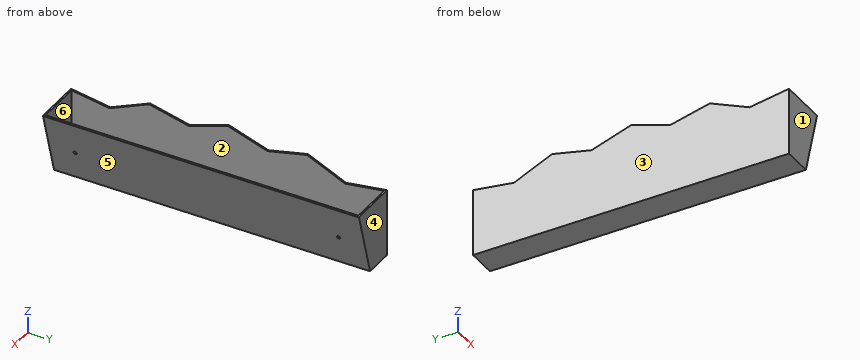
from build123d import *

# Parameters (mm, degrees)
F1_DEPTH  = 304.8
F4_DEPTH  = 1.5875
F6_DEPTH  = 1.5875
F8_DEPTH  = 25.4
F9_DEPTH  = 25.4
F10_DEPTH = 1.5875


with BuildPart() as f1:
    # F0 (on Front) → F1 (new body)
    with BuildSketch(Plane.XZ):
        Polygon((0, 0), (0, 63.5), (-1.5875, 63.5), (-1.5875, -1.5875), (26.5975192948, -1.5875), (45.0656705162, 63.0639608604), (43.5392282085, 63.5), (25.4, 0), align=None)
    extrude(amount=F1_DEPTH)

    # F3 (on face) → F4 (join)
    with BuildSketch(Plane.XZ.offset(304.8)):
        Polygon((43.5392282085, 63.5), (0, 63.5), (0, 0), (25.4, 0), align=None)
    extrude(amount=-F4_DEPTH)

    # F5 (on face) → F6 (join)
    with BuildSketch(Plane(origin=(0, 0, 0), x_dir=(-1, 0, 0), z_dir=(0, 1, 0))):
        Polygon((0, 63.5), (-43.5392282085, 63.5), (-25.4, 0), (0, 0), align=None)
    extrude(amount=-F6_DEPTH)

    # F7 (on face) → F8 (cut)
    with BuildSketch(Plane(origin=(25.0101701183, 0, -7.1443335954), x_dir=(0, 1, 0), z_dir=(0.9615384615, 0, -0.2746703242))):
        with BuildLine():
            ThreePointArc((-279.4, 35.9416069393), (-278.2774679849, 36.4065749241), (-277.8125, 37.5291069393))
            ThreePointArc((-277.8125, 37.5291069393), (-279.4, 39.1166069393), (-280.9875, 37.5291069393))
            ThreePointArc((-280.9875, 37.5291069393), (-280.5225320151, 36.4065749241), (-279.4, 35.9416069393))
        make_face()
        with BuildLine():
            ThreePointArc((-23.8125, 37.5291069393), (-26.5225320151, 38.6516389544), (-25.4, 35.9416069393))
            ThreePointArc((-25.4, 35.9416069393), (-24.2774679849, 36.4065749241), (-23.8125, 37.5291069393))
        make_face()
    extrude(amount=-F8_DEPTH, mode=Mode.SUBTRACT)

    # F2 (on face) → F9 (cut)
    with BuildSketch(Plane.YZ):
        Polygon((-52.2120932715, 63.5), (-39.4870413326, 57.779973409), (-0.1351656424, 63.5), align=None)
        Polygon((-304.8, 63.5), (-266.746729324, 57.5579500411), (-253.1458196474, 63.5), align=None)
    extrude(amount=-F9_DEPTH, mode=Mode.SUBTRACT)

    # F2 (on face) → F10 (join)
    with BuildSketch(Plane.YZ):
        Polygon((-0.1351656424, 63.5), (-39.4870413326, 57.779973409), (0, 63.5), align=None)
        with BuildLine():
            Line((-76.2, 50.6074602206), (0, 50.6074602206))
            ThreePointArc((0, 50.6074602206), (-19.6950538014, 54.4605428278), (-39.4870413326, 57.779973409))
            ThreePointArc((-39.4870413326, 57.779973409), (-57.8141368142, 60.3662538666), (-76.2, 62.4949413282))
            Line((-76.2, 62.4949413282), (-76.2, 50.6074602206))
        make_face()
        with BuildLine():
            Line((-152.4, 50.6074602206), (-76.2, 50.6074602206))
            Line((-76.2, 50.6074602206), (-76.2, 62.4949413282))
            ThreePointArc((-76.2, 62.4949413282), (-81.4321305003, 63.0160017697), (-86.6678194969, 63.5))
            Line((-86.6678194969, 63.5), (-152.4, 63.5))
            Line((-152.4, 63.5), (-152.4, 50.6074602206))
        make_face()
        with BuildLine():
            ThreePointArc((-76.2, 62.4949413282), (-57.8141368142, 60.3662538666), (-39.4870413326, 57.779973409))
            Line((-39.4870413326, 57.779973409), (-52.2120932715, 63.5))
            Line((-52.2120932715, 63.5), (-76.2, 74.2827822634))
            Line((-76.2, 74.2827822634), (-114.3780665248, 65.4410439145))
            ThreePointArc((-114.3780665248, 65.4410439145), (-100.5138654868, 64.6001122426), (-86.6678194969, 63.5))
            Line((-86.6678194969, 63.5), (-76.2, 63.5))
            Line((-76.2, 63.5), (-76.2, 62.4949413282))
        make_face()
        with BuildLine():
            Line((-228.693458648, 50.6074602206), (-152.4, 50.6074602206))
            Line((-152.4, 50.6074602206), (-152.4, 63.5))
            Line((-152.4, 63.5), (-152.4, 66.4151452364))
            ThreePointArc((-152.4, 66.4151452364), (-171.4790500008, 66.1699929381), (-190.545501947, 65.4346979192))
            ThreePointArc((-190.545501947, 65.4346979192), (-209.6384806919, 64.2057492114), (-228.693458648, 62.4852936405))
            Line((-228.693458648, 62.4852936405), (-228.693458648, 50.6074602206))
        make_face()
        with BuildLine():
            Line((-266.746729324, 50.6074602206), (-228.693458648, 50.6074602206))
            Line((-228.693458648, 50.6074602206), (-228.693458648, 62.4852936405))
            ThreePointArc((-228.693458648, 62.4852936405), (-247.7519270715, 60.2674648579), (-266.746729324, 57.5579500411))
            Line((-266.746729324, 57.5579500411), (-266.746729324, 50.6074602206))
        make_face()
        with BuildLine():
            Line((-152.4, 66.4151452364), (-152.4, 63.5))
            Line((-152.4, 63.5), (-86.6678194969, 63.5))
            ThreePointArc((-86.6678194969, 63.5), (-100.5138654868, 64.6001122426), (-114.3780665248, 65.4410439145))
            ThreePointArc((-114.3780665248, 65.4410439145), (-133.3827952989, 66.1715799592), (-152.4, 66.4151452364))
        make_face()
        with BuildLine():
            Line((-304.8, 50.6074602206), (-266.746729324, 50.6074602206))
            Line((-266.746729324, 50.6074602206), (-266.746729324, 57.5579500411))
            ThreePointArc((-266.746729324, 57.5579500411), (-285.818633363, 54.3305469631), (-304.8, 50.6074602206))
        make_face()
        with BuildLine():
            ThreePointArc((-266.746729324, 57.5579500411), (-247.7519270715, 60.2674648579), (-228.693458648, 62.4852936405))
            ThreePointArc((-228.693458648, 62.4852936405), (-209.6384806919, 64.2057492114), (-190.545501947, 65.4346979192))
            Line((-190.545501947, 65.4346979192), (-228.4648343576, 74.2827822634))
            Line((-228.4648343576, 74.2827822634), (-266.746729324, 57.5579500411))
        make_face()
        with BuildLine():
            Line((-152.4, 77.841184886), (-152.4, 66.4151452364))
            ThreePointArc((-152.4, 66.4151452364), (-133.3827952989, 66.1715799592), (-114.3780665248, 65.4410439145))
            Line((-114.3780665248, 65.4410439145), (-152.4, 77.841184886))
        make_face()
        with BuildLine():
            ThreePointArc((-190.545501947, 65.4346979192), (-171.4790500008, 66.1699929381), (-152.4, 66.4151452364))
            Line((-152.4, 66.4151452364), (-152.4, 77.841184886))
            Line((-152.4, 77.841184886), (-190.545501947, 65.4346979192))
        make_face()
    extrude(amount=-F10_DEPTH)


solid = f1.part
Can you work these out from the model? Positions are in its coordinate system, mm. Face numbers are marked on the shaded views. A direction names the side the tool comes from. Give positions to 0.01 mm unless a question says otherwise; leave off trailing zeros. Order: outer loops, then holes, each group sorted by start corner. A loop starts at its lowest first (then second) coordinate and runs counter-clockwise, first axis right, second up. Notation, with made-up numbers: M 10,20 L 67,20 A22 cw 67,32 Z; hole C 1.5,-11 d10. An arc over 180 degrees is marked long. Use a Markdown table: item, result. Add a question column.
Item 1: Will these pins go through, and if not, where does the flat tip stop? pin 1 (12 mm diameter, centred on x = 37, z = 67.5, fed in from +Y); pin 2 (6 mm diameter, centred on x = 18, y = -92.5, fed in from +Z); pin 3 (6 mm diameter, centred on y = -198.5, z = 16, fed in from +X); pin 4 (23.5 mm diameter, centred on y = -201.5, z = 31, fed in from +X).
Item 2: If I drill on L1, parallel to Y at x = 30, z = 17.5; L2, parallel to X at y = -204.5, z = 6.5; L3, parallel to X at y = -105.5, z = 12, over which ranges is the centre line in solid material (lowest first)? Write a range as [from, to].
Item 3: Suppose I cut it at A-A (x = 11). List the corners of the cut face in (y, z) for me.
Item 4: Suppose I cut it at B-B (z = 43). List the corners of the cut face in (x, y) for me, then the cut area to 3 significant figures.
Item 5: For the marked faces 1 and 2, which set-ups out of +Z, -Z, +X, -X, +Y, -Y let a thin tool reach every point of the face, with its end or its side?
Item 6: We'd pull the mould along X, two halves only. Please class the marked faces 3, 4, 5 and 6: +X half, -X half, draft (parallel to the pull), parting line (faces both ways), or undercut.
Item 7: Suppose I cut it at D-D (z = 14.5). List the corners of the cut face in (x, y) for me, then the cut area to 3 significant figures.
Item 8: Suppose I cut it at C-C (y = -174.5). List the corners of the cut face in (x, z) for me, then the cut area to 3 significant figures.
Answer sheet:
| question | item | result |
|---|---|---|
| 1 | pin 1 | stops at y = 0 |
| 1 | pin 2 | stops at z = 0 |
| 1 | pin 3 | stops at x = 32.48 |
| 1 | pin 4 | stops at x = 39.26 |
| 2 | L1 | y = [-304.8, -303.21], [-1.59, 0] |
| 2 | L2 | x = [-1.59, 0], [27.26, 28.91] |
| 2 | L3 | x = [-1.59, 0], [28.83, 30.48] |
| 3 | outline | M -304.8,-1.59 L 0,-1.59 L 0,63.5 L -1.59,63.5 L -1.59,0 L -303.21,0 L -303.21,63.5 L -304.8,63.5 Z |
| 4 | outline | M -1.59,-304.8 L 39.33,-304.8 L 39.33,0 L -1.59,0 Z; hole M 0,-303.21 L 37.68,-303.21 L 37.68,-1.59 L 0,-1.59 Z |
| 4 | area | 1,110 mm² |
| 5 | face 1 | +Z, -Z, +X, -X, -Y |
| 5 | face 2 | +Z |
| 6 | face 3 | -X half |
| 6 | face 4 | draft |
| 6 | face 5 | +X half |
| 6 | face 6 | undercut |
| 7 | outline | M -1.59,-304.8 L 31.19,-304.8 L 31.19,0 L -1.59,0 Z; hole M 0,-303.21 L 29.54,-303.21 L 29.54,-1.59 L 0,-1.59 Z |
| 7 | area | 1,080 mm² |
| 8 | outline | M -1.59,-1.59 L 26.6,-1.59 L 45.07,63.06 L 43.54,63.5 L 25.4,0 L 0,0 L 0,70.65 L -1.59,70.65 Z |
| 8 | area | 262 mm² |
